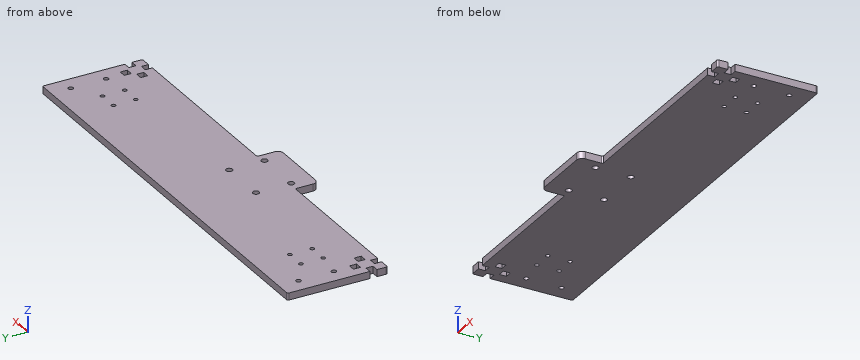
```python
from build123d import *

# Parameters (mm, degrees)
SKETCH1_R           = 1.5
SKETCH1_R_2         = 1.75
SKETCH1_R_3         = 2.25
SKETCH1_W           = 5
SKETCH1_H           = 5
BOSS_EXTRUDE1_DEPTH = 5


with BuildPart() as part:
    # Sketch1 → Boss-Extrude1 (new body)
    with BuildSketch(Plane.XY):
        with BuildLine():
            Line((-10, -2.501863855), (-10, -9.001863855))
            ThreePointArc((-10, -9.001863855), (-9.707106781, -9.708970637), (-9, -10.001863855))
            Line((-9, -10.001863855), (-2.5, -10.001863855))
            Line((-2.5, -10.001863855), (-2.5, -5.001863855))
            Line((-2.5, -5.001863855), (2.5, -5.001863855))
            Line((2.5, -5.001863855), (2.5, -10.001863855))
            Line((2.5, -10.001863855), (105.724043242, -10.001863855))
            ThreePointArc((105.724043242, -10.001863855), (106.431150023, -10.294757074), (106.724043242, -11.001863855))
            Line((106.724043242, -11.001863855), (106.724043242, -22.458474266))
            ThreePointArc((106.724043242, -22.458474266), (107.895616117, -25.286901391), (110.724043242, -26.458474266))
            Line((110.724043242, -26.458474266), (151.039811852, -26.458474266))
            ThreePointArc((151.039811852, -26.458474266), (153.868238976, -25.286901391), (155.039811852, -22.458474266))
            Line((155.039811852, -22.458474266), (155.039811852, -11.001863855))
            ThreePointArc((155.039811852, -11.001863855), (155.33270507, -10.294757074), (156.039811852, -10.001863855))
            Line((156.039811852, -10.001863855), (287.5, -10.001863855))
            Line((287.5, -10.001863855), (287.5, -5.001863855))
            Line((287.5, -5.001863855), (292.5, -5.001863855))
            Line((292.5, -5.001863855), (292.5, -10.001863855))
            Line((292.5, -10.001863855), (299, -10.001863855))
            ThreePointArc((299, -10.001863855), (299.707106781, -9.708970637), (300, -9.001863855))
            Line((300, -9.001863855), (300, -2.501863855))
            Line((300, -2.501863855), (295, -2.501863855))
            Line((295, -2.501863855), (295, 2.498136145))
            Line((295, 2.498136145), (300, 2.498136145))
            Line((300, 2.498136145), (300, 60))
            ThreePointArc((300, 60), (299.707106781, 60.707106781), (299, 61))
            Line((299, 61), (-9, 61))
            ThreePointArc((-9, 61), (-9.707106781, 60.707106781), (-10, 60))
            Line((-10, 60), (-10, 2.498136145))
            Line((-10, 2.498136145), (-5, 2.498136145))
            Line((-5, 2.498136145), (-5, -2.501863855))
            Line((-5, -2.501863855), (-10, -2.501863855))
        make_face()
        with Locations((33.4, 34.947207957)):
            Circle(SKETCH1_R, mode=Mode.SUBTRACT)
        with Locations((19.5, 34.947207957)):
            Circle(SKETCH1_R, mode=Mode.SUBTRACT)
        with Locations((256.6, 34.947207957)):
            Circle(SKETCH1_R, mode=Mode.SUBTRACT)
        with Locations((270.5, 34.947207957)):
            Circle(SKETCH1_R, mode=Mode.SUBTRACT)
        with Locations((270.5, 19.147207957)):
            Circle(SKETCH1_R, mode=Mode.SUBTRACT)
        with Locations((256.6, 19.147207957)):
            Circle(SKETCH1_R, mode=Mode.SUBTRACT)
        with Locations((289, 22.001504258)):
            Circle(SKETCH1_R_2, mode=Mode.SUBTRACT)
        with Locations((19.5, 19.147207957)):
            Circle(SKETCH1_R, mode=Mode.SUBTRACT)
        with Locations((148.082820817, 13.683948234)):
            Circle(SKETCH1_R_3, mode=Mode.SUBTRACT)
        with Locations((148.082820817, -11.316051766)):
            Circle(SKETCH1_R_3, mode=Mode.SUBTRACT)
        with Locations((289, 47.001504258)):
            Circle(SKETCH1_R_2, mode=Mode.SUBTRACT)
        with Locations((1, 22.001504258)):
            Circle(SKETCH1_R_2, mode=Mode.SUBTRACT)
        with Locations((1, 47.001504258)):
            Circle(SKETCH1_R_2, mode=Mode.SUBTRACT)
        with Locations((33.4, 19.147207957)):
            Circle(SKETCH1_R, mode=Mode.SUBTRACT)
        with Locations((114.224914373, -11.316051766)):
            Circle(SKETCH1_R_3, mode=Mode.SUBTRACT)
        with Locations((114.224914373, 13.683948234)):
            Circle(SKETCH1_R_3, mode=Mode.SUBTRACT)
        with Locations((0, 7.498136145)):
            Rectangle(SKETCH1_W, SKETCH1_H, mode=Mode.SUBTRACT)
        with Locations((7.5, -0.001863855)):
            Rectangle(SKETCH1_W, SKETCH1_H, mode=Mode.SUBTRACT)
        with Locations((282.5, -0.001863855)):
            Rectangle(SKETCH1_W, SKETCH1_H, mode=Mode.SUBTRACT)
        with Locations((290, 7.498136145)):
            Rectangle(SKETCH1_W, SKETCH1_H, mode=Mode.SUBTRACT)
    extrude(amount=BOSS_EXTRUDE1_DEPTH)


solid = part.part
```
Model file for the job. Use its own axes, mm. Coordinates: 2 decimals unless noted, no trailing zeros. Order: outer loops, then holes, each group sorted by start corner. A loop starts at its lowest first (then second) coordinate and runs counter-clockwise, first axis right, second up. Notation, with made-up numbers: (19.25, 37) -> (49.25, 37) arc R12 ccw to (49.25, 53) -> close; hole circle Ø11 at (65, -16.5). An arc over 180 degrees is marked (long way). Return JSON: item names as keys, results as strings.
Item 1: Pin check, flat tips, straight feed: P1, Ø10, axis at x = 86.5, y = 36, coming from the -Z side; P2, Ø1.5, axis at x = 290.5, z = 2, coming from the -Y side; P3, Ø2.5, axis at x = 66.5, z = 1.5, coming from the -Y side; P4, Ø1.5, axis at y = -1, z = 2, coming from the +X side. Stop position of each tip, or through.
Model answer:
{"P1": "stops at z = 0", "P2": "stops at y = -5", "P3": "stops at y = -10", "P4": "stops at x = 295"}
Item 2: Slice it at A-A (x = 168). Write the cut outline in (y, z), then the cut area to 3 significant figures.
Model answer:
{"outline": "(-10, 0) -> (61, 0) -> (61, 5) -> (-10, 5) -> close", "area": "355 mm²"}
Item 3: Wall check: line 1 along X through (y, z) = (8, 1.75); line 2 along Y through (x, z) = (19.5, 3.5); line 3 along X through (y, z) = (13.5, 1.55). Give the ranges that are in metal, low to high. Write a range as from..to.
Model answer:
{"line 1": "x = -10..-2.5, 2.5..287.5, 292.5..300", "line 2": "y = -10..17.65, 20.65..33.45, 36.45..61", "line 3": "x = -10..111.98, 116.47..145.84, 150.33..300"}
Item 4: Slice it at B-B (z = 1.4). Count the separate pieces of the cut face and the enclosed holes in it, then the cut area to 3 significant figures.
Model answer:
{"separate pieces": "1", "enclosed holes": "20", "area": "22,400 mm²"}
